from build123d import *

# Parameters (mm, degrees)
F0_W      = 50.8
F0_H      = 114.3
F1_DEPTH  = 12.7
F2_R      = 8.89
F3_DEPTH  = 63.5
F4_W      = 25.4
F4_H      = 50.8
F5_DEPTH  = 27.94
F8_DEPTH  = 12.7
F9_DEPTH  = 12.7
F10_R     = 3.175
F11_DEPTH = 76.2
F12_W     = 25.4
F12_H     = 15.24
F13_DEPTH = 76.2


with BuildPart() as f1:
    # F0 (on Top) → F1 (new body, symmetric)
    with BuildSketch(Plane.XY):
        with BuildLine():
            Line((-25.4, 57.15), (25.4, 57.15))
            ThreePointArc((25.4, 57.15), (0, 82.55), (-25.4, 57.15))
        make_face()
        Rectangle(F0_W, F0_H)
        with BuildLine():
            ThreePointArc((-25.4, -57.15), (0, -82.55), (25.4, -57.15))
            Line((25.4, -57.15), (-25.4, -57.15))
        make_face()
    extrude(amount=F1_DEPTH, both=True)

    # F2 (on face) → F3 (cut)
    with BuildSketch(Plane.XY.offset(12.7)):
        with Locations((0, 55.88)):
            Circle(F2_R)
        with Locations((0, -55.88)):
            Circle(F2_R)
    extrude(amount=-F3_DEPTH, mode=Mode.SUBTRACT)

    # F4 (on face) → F5 (join)
    with BuildSketch(Plane.XY.offset(12.7)):
        Rectangle(F4_W, F4_H)
    extrude(amount=F5_DEPTH)

    # F7 (on face) → F8 (join)
    with BuildSketch(Plane.XZ.offset(25.4)):
        with BuildLine():
            Line((-12.7, 40.64), (12.7, 40.64))
            ThreePointArc((12.7, 40.64), (0, 53.34), (-12.7, 40.64))
        make_face()
    extrude(amount=-F8_DEPTH)

    # F6 (on face) → F9 (join)
    with BuildSketch(Plane(origin=(0, 25.4, 0), x_dir=(-1, 0, 0), z_dir=(0, 1, 0))):
        with BuildLine():
            Line((-12.7, 40.64), (12.7, 40.64))
            ThreePointArc((12.7, 40.64), (0, 53.34), (-12.7, 40.64))
        make_face()
    extrude(amount=-F9_DEPTH)

    # F10 (on face) → F11 (cut)
    with BuildSketch(Plane.XZ.offset(25.4)):
        with Locations((0, 45.72)):
            Circle(F10_R)
    extrude(amount=-F11_DEPTH, mode=Mode.SUBTRACT)

    # F12 (on face) → F13 (cut)
    with BuildSketch(Plane.YZ.offset(12.7)):
        with Locations((0, 33.02)):
            Rectangle(F12_W, F12_H)
        with BuildLine():
            ThreePointArc((-12.7, 25.4), (0, 17.249871), (12.7, 25.4))
            Line((12.7, 25.4), (-12.7, 25.4))
        make_face()
    extrude(amount=-F13_DEPTH, mode=Mode.SUBTRACT)


solid = f1.part
Can you work these out from the model? Positions are in its coordinate system, mm. A direction names the side the tool comes from. Coordinates: 2 decimals unless noted, no trailing zeros. Loops run counter-clockwise (first coordinate to the right, second up) from the corner with the lowest first, then second, coordinate; pieces in that order, holes last. Notation, with made-up numbers: (-33.5, 69) - (24.5, 69) arc R30 cw to (24.5, 106) - close; hole circle Ø5 at (-38, 81). An arc over 180 degrees is marked (long way). Answer as a JSON object with one key per item and string values. Group by question number.
Item 1: If we section it at A-A (z = 32.5): List the corners of the cut face in (x, y) for me, plus the area to 3 significant figures.
Item 2: For pin 1 (2 mm diameter, centred on x = -16.5, y = -24.5, fed in from +Z); pin 2 (12.5 mm diameter, centred on x = 5, z = 39.5, fed in from -Y); pin 3 (12 mm diameter, centred on y = -16, z = 29, fed in from -X); pin 4 (4 mm diameter, centred on x = 16.5, z = 27.5, fed in from -Y), each with a flat end and sliding along its axis, tell me the tip position at first contact or that it passes through.
Item 3: If we section it at B-B (z = 45.72): List the corners of the cut face in (x, y) for me (3 decimals).
Item 4: If we section it at D-D (z = 11): List the corners of the cut face in (x, y) for me.
Item 5: If we mould it in two halves opening along X, with no side actions, what happens to faces 4 (the face through (0, 25.4, 33)), 5 (the face through (1.7, -19.1, 48.4)), 6 (the face through (-1.93, -64.56, 0.18)), 7 (the face through (0.279, -19.139, 53.337))? For each: released by +X, released by -X, zero draft, split by the parting line, or undercut.
Item 6: On a 3-axis mill with a long thin cutter (end or side, diameter ignored), from which of +Z, -Z, +X, -X, +Y, -Y can I reach the whole of each face in a straight line? I mean faces 1 (the face through (12.7, 0, 17)), 2 (the face through (0, -25.4, 33)), 3 (the face through (0, 12.7, 36)). Say none if no direction works.
Item 7: If we section it at C-C (y = -7): List the corners of the cut face in (x, z) for me, plus the area to 3 significant figures.
Item 8: If I drill on L1, parallel to Y at x = 0, z = -0.5; L2, parallel to Z at x = 0, y = -15 (3 decimals); L3, parallel to Z at x = 9, y = -48.5, over which ranges is the centre line in solid material (lowest first)? Write a range as from..to.
Returned:
{
 "1": {"outline": "(-12.7, -25.4) - (12.7, -25.4) - (12.7, -12.7) - (-12.7, -12.7) - close; (-12.7, 12.7) - (12.7, 12.7) - (12.7, 25.4) - (-12.7, 25.4) - close", "area": "645 mm²"},
 "2": {"pin 1": "stops at z = 12.7", "pin 2": "stops at y = -25.4", "pin 3": "stops at x = -12.7", "pin 4": "passes through"},
 "3": {"outline": "(-11.64, -25.4) - (-3.175, -25.4) - (-3.175, -12.7) - (-11.64, -12.7) - close; (-11.64, 12.7) - (-3.175, 12.7) - (-3.175, 25.4) - (-11.64, 25.4) - close; (3.175, -25.4) - (11.64, -25.4) - (11.64, -12.7) - (3.175, -12.7) - close; (3.175, 12.7) - (11.64, 12.7) - (11.64, 25.4) - (3.175, 25.4) - close"},
 "4": {"outline": "(-25.4, -57.15) arc R25.4 ccw to (25.4, -57.15) - (25.4, 57.15) arc R25.4 ccw to (-25.4, 57.15) - close; hole circle Ø17.78 at (0, -55.88); hole circle Ø17.78 at (0, 55.88)"},
 "5": {"face 4": "zero draft", "face 5": "undercut", "face 6": "undercut", "face 7": "split by the parting line"},
 "6": {"face 1": "+Z, +X, +Y, -Y", "face 2": "+Z, +X, -X, -Y", "face 3": "+Z, +X, -X"},
 "7": {"outline": "(-25.4, -12.7) - (25.4, -12.7) - (25.4, 12.7) - (12.7, 12.7) - (12.7, 19.13) - (-12.7, 19.13) - (-12.7, 12.7) - (-25.4, 12.7) - close", "area": "1,450 mm²"},
 "8": {"L1": "y = -82.55..-64.77, -46.99..46.99, 64.77..82.55", "L2": "z = -12.7..42.545, 48.895..53.34", "L3": "z = -12.7..12.7"}
}
